```python
from build123d import *

# Parameters (mm, degrees)
SKETCH1_R           = 250
SKETCH1_R_2         = 162.5
BOSS_EXTRUDE1_DEPTH = 19
SKETCH2_R           = 215
SKETCH2_R_2         = 192.5
CUT_EXTRUDE1_DEPTH  = 7
SKETCH3_R           = 5
CUT_EXTRUDE2_DEPTH  = 355.063553617


with BuildPart() as part:
    # Sketch1 → Boss-Extrude1 (new body)
    with BuildSketch(Plane(origin=(0, 0, 0), x_dir=(1, 0, 0), z_dir=(0, 1, 0))):
        with Locations(Location((0, 0, 0), (0, 0, 270))):
            Circle(SKETCH1_R)
        with Locations(Location((0, 0, 0), (0, 0, 270))):
            Circle(SKETCH1_R_2, mode=Mode.SUBTRACT)
    extrude(amount=BOSS_EXTRUDE1_DEPTH)

    # Sketch2 → Cut-Extrude1 (cut)
    with BuildSketch(Plane(origin=(0, 19, 0), x_dir=(1, 0, 0), z_dir=(0, 1, 0))):
        with Locations(Location((0, 0, 0), (0, 0, 270))):
            Circle(SKETCH2_R)
        with Locations(Location((0, 0, 0), (0, 0, 270))):
            Circle(SKETCH2_R_2, mode=Mode.SUBTRACT)
    extrude(amount=-CUT_EXTRUDE1_DEPTH, mode=Mode.SUBTRACT)

    # Sketch3 → Cut-Extrude2 (cut, through all)
    with BuildSketch(Plane.XZ):
        with Locations(Location((111.25, 192.690652342, 0), (0, 0, 270))):
            Circle(SKETCH3_R)
        with Locations(Location((222.5, 0, 0), (0, 0, 270))):
            Circle(SKETCH3_R)
        with Locations(Location((-222.5, 0, 0), (0, 0, 90))):
            Circle(SKETCH3_R)
        with Locations(Location((-111.25, 192.690652342, 0), (0, 0, 90))):
            Circle(SKETCH3_R)
        with Locations(Location((111.25, -192.690652342, 0), (0, 0, 90))):
            Circle(SKETCH3_R)
        with Locations(Location((-111.25, -192.690652342, 0), (0, 0, 270))):
            Circle(SKETCH3_R)
    extrude(amount=-CUT_EXTRUDE2_DEPTH, mode=Mode.SUBTRACT)


solid = part.part
```
Geometry check sheet. Reference: the model listing, model coordinates, mm. A direction names the side the tool comes from. Coordinates: 2 decimals unless noted, no trailing zeros. Order: outer loops, then holes, each group sorted by start corner. A loop starts at its lowest first (then second) coordinate and runs counter-clockwise, first axis right, second up.
Item 1: Section check B-B (z = 68). Enter the section's corners in (x, y).
Item 2: Section check A-A (x = 0). Enter the section's corners in (y, z).
Item 3: Depth check by flat-ended pin: pin 1 (13 mm diameter, centred on x = -111.25, z = -192.69, fed in from -Y); pin 2 (1 mm diameter, centred on x = 32.5, y = 9.5, fed in from +Z); pin 3 (10 mm diameter, centred on x = -32, y = 13, fed in from +Z); pin 4 (8 mm diameter, centred on x = 153.5, y = 7, fed in from -Z). Enter the tip coordinate at first touch or a pass-through.
Item 4: Mould release check, pull along X, two halves, no side actions. Record for faces 1 (the cylindrical face through (10.99, 9.37, -249.76)), 2 (the flat face through (-203, 19, 73)), 3 (the cylindrical face through (-209.887, 15.549, -46.608)): released by +X, released by -X, zero draft, split by the parting line, or undercut.
Item 5: Section check C-C (x = -176.5). Enter the section's corners in (y, z), plus the area to 3 significant figures.
Item 6: Tool access check on faces 4 (the flat face through (-110, 12, -160)), 5 (the cylindrical face through (137.02, 9.37, 87.36)). Record the directions out of +Z, -Z, +X, -X, +Y, -Y that give a thin tool (end or side, any length) a straight path to the whole face; none if there is none.
Item 7: Scan lines: line 1 along X through (y, z) = (10.5, 0); line 2 along X through (y, z) = (14, 0); line 3 along X through (y, z) = (5, 196.5). Record each from-to range of solid material in increasing order.
Check sheet entries:
1. outline: (-240.57, 0) - (-147.59, 0) - (-147.59, 19) - (-180.09, 19) - (-180.09, 12) - (-203.96, 12) - (-203.96, 19) - (-240.57, 19) - close; (147.59, 0) - (240.57, 0) - (240.57, 19) - (203.96, 19) - (203.96, 12) - (180.09, 12) - (180.09, 19) - (147.59, 19) - close
2. outline: (0, -250) - (19, -250) - (19, -215) - (12, -215) - (12, -192.5) - (19, -192.5) - (19, -162.5) - (0, -162.5) - close; (0, 162.5) - (19, 162.5) - (19, 192.5) - (12, 192.5) - (12, 215) - (19, 215) - (19, 250) - (0, 250) - close
3. pin 1: stops at y = 0
3. pin 2: stops at z = 247.94
3. pin 3: stops at z = 248.54
3. pin 4: stops at z = -200.37
4. face 1: split by the parting line
4. face 2: zero draft
4. face 3: undercut
5. outline: (0, -177.05) - (19, -177.05) - (19, -122.77) - (12, -122.77) - (12, -76.84) - (19, -76.84) - (19, 76.84) - (12, 76.84) - (12, 122.77) - (19, 122.77) - (19, 177.05) - (0, 177.05) - close
5. area: 6,080 mm2
6. face 4: +Y
6. face 5: +Y, -Y
7. line 1: x = -250 to -227.5, -217.5 to -162.5, 162.5 to 217.5, 227.5 to 250
7. line 2: x = -250 to -227.5, -217.5 to -215, -192.5 to -162.5, 162.5 to 192.5, 215 to 217.5, 227.5 to 250
7. line 3: x = -154.56 to -114.49, -108.01 to 108.01, 114.49 to 154.56
